The listing builds one solid part. Answer for the finished solid, in the listing's coordinates (mm). A direction names the side the tool comes from. Coordinates: 2 decimals unless noted, no trailing zeros. Write each loop counter-clockwise with the first axis right and the second up, starting at its lowest first coordinate (ties: lowest second). Pieces come first, ordered by that corner, then holes. Notation, with made-up numbers: M 81,74.5 L 131,74.5 A16 ccw 131,103.5 Z; hole C 0,57 d3. An arc over 180 degrees is marked long. Answer as CSV lines item,"result".
```python
from build123d import *

# Parameters (mm, degrees)
BOSS_EXTRUDE1_DEPTH            = 4.7625
SKETCH5_R                      = 10
CUT_EXTRUDE1_DEPTH             = 90.919995629
M8_CLEARANCE_HOLE1_D           = 9
FILLET1_R                      = 25
M5_CLEARANCE_HOLE1_D           = 5.5
M5_CLEARANCE_HOLE1_CSINK_D     = 5.55
M5_CLEARANCE_HOLE1_CSINK_ANGLE = 90
FILLET2_R                      = 5


with BuildPart() as part:
    # Sketch1 → Boss-Extrude1 (new body)
    with BuildSketch(Plane(origin=(0, 0, 0), x_dir=(1, 0, 0), z_dir=(0, 1, 0))):
        with BuildLine():
            Line((-12.5, -82.691742077), (12.5, -82.691742077))
            Line((12.5, -82.691742077), (12.5, -32.691742077))
            ThreePointArc((12.5, -32.691742077), (0, 35), (-12.5, -32.691742077))
            Line((-12.5, -32.691742077), (-12.5, -82.691742077))
        make_face()
    extrude(amount=BOSS_EXTRUDE1_DEPTH)

    # Sketch5 → Cut-Extrude1 (cut, through all)
    with BuildSketch(Plane.XZ):
        with Locations(Location((0, 0, 0), (0, 0, 270))):
            Circle(SKETCH5_R)
    extrude(amount=-CUT_EXTRUDE1_DEPTH, mode=Mode.SUBTRACT)

    # M8 Clearance Hole1 (through all)
    with Locations(Plane(origin=(0, 0, 0), x_dir=(-1, 0, 0), z_dir=(0, -1, 0))):
        with Locations((0, -47.691742077), (0, -72.691742077)):
            Hole(M8_CLEARANCE_HOLE1_D / 2)

    # Fillet1
    fillet1_edges = [part.edges().sort_by_distance(p)[0] for p in [
        (-12.5, 2.38125, 32.691742077),
        (12.5, 2.38125, 32.691742077),
    ]]
    fillet(fillet1_edges, radius=FILLET1_R)

    # M5 Clearance Hole1 (through all)
    with Locations(Plane(origin=(0, 0, 0), x_dir=(-1, 0, 0), z_dir=(0, -1, 0))):
        with Locations((-12, 24), (8, 24), (-26, 10), (-26, -10), (-12, -24), (8, -24)):
            CounterSinkHole(M5_CLEARANCE_HOLE1_D / 2, M5_CLEARANCE_HOLE1_CSINK_D / 2, counter_sink_angle=M5_CLEARANCE_HOLE1_CSINK_ANGLE)

    # Fillet2
    fillet2_edges = [part.edges().sort_by_distance(p)[0] for p in [
        (12.5, 2.38125, 82.691742077),
        (-12.5, 2.38125, 82.691742077),
    ]]
    fillet(fillet2_edges, radius=FILLET2_R)


solid = part.part
```
Q1. A flat-ended cylindrical pin translates along its axis: pin 1 Ø4.5 at (x, z) = (26, 10) entering from -Y. Find the tip coordinate at first contact, or state that the pin passes through.
Output:
pin 1,"through"
Q2. Find section A-A (z = 0). Give the vertices of the cut face in (x, y), and give its area (3 significant figures).
Output:
outline,"M -35,0 L -10,0 L -10,4.76 L -35,4.76 Z; M 10,0 L 35,0 L 35,4.76 L 10,4.76 Z"
area,"238 mm2"
Q3. The mould has two halves that part along X. Classify faces 1 (the flat face through (-12.5, 2, 62)), 2 (the flat face through (7, 0, 10)), 3 (the cylindrical face through (-0.976, 2.415, 52.085)): pulls with the +X half, pulls with the -X half, needs draft (parallel to the pull), parting line crosses it, or undercut.
Output:
face 1,"pulls with the -X half"
face 2,"needs draft"
face 3,"undercut"
Q4. Find section D-D (z = -17). Give the vertices of the cut face in (x, y), and give its area (3 significant figures).
Output:
outline,"M -30.59,0 L 30.59,0 L 30.59,4.76 L -30.59,4.76 Z"
area,"291 mm2"
Q5. For faces 4 (the flat face through (12.5, 2, 62)), 5 (the cylindrical face through (-11.07, 2.41, 81.19)), determine the directions among +Z, -Z, +X, -X, +Y, -Y from which every point of the face is accessible in a straight line to the end or side of a thin tool.
Output:
face 4,"+Z, +X, +Y, -Y"
face 5,"+Z, -X, +Y, -Y"
Q6. Find section B-B (x = 26). Count the separate pieces of the cut face and the enclosed holes in it, and give its area (3 significant figures).
Output:
separate pieces,"3"
enclosed holes,"0"
area,"171 mm2"
Q7. Straight lines are drawn through the part: line 1 (Z direction, x = -0.5, y = 0.6); line 2 (X direction, y = 0.5, z = -22.5); line 3 (Z direction, x = 24.5, y = 1.35) (3 decimals). For each, find the intervals that lie inside material, in ascending order.
Output:
line 1,"-35 to -9.99, 9.99 to 43.22, 52.16 to 68.22, 77.16 to 82.69"
line 2,"-26.81 to -10.3, -5.7 to 9.7, 14.3 to 26.81"
line 3,"-24.995 to -12.305, -7.695 to 7.695, 12.305 to 24.995"
